The drawing under review shows one solid part. Ordinate dimensions are in mm from its lowest x, y, z. Give positions to 0.01 mm unless a question says otherwise; leave off trailing zeros. Loops run counter-clockwise (first coordinate to the right, second up) from the corner with the lowest first, then second, coordinate; pieces in that order, holes last. Notation, with made-up numbers: M 24.25,54 L 59.25,54 A6 cw 59.25,65 Z; hole C 9,31 d10. An arc over 180 degrees is marked long. One line per item, written item: value. Start each with the question number.
Q1. We need section B-B on y = 3.5. Write out the cut boundary in (x, z), plus the area to 3 significant figures.
Q2. For pin 1 (1.5 mm diameter, centred on y = 36.5, z = 30.5, fed in from -X); pin 2 (3 mm diameter, centred on x = 193.5, y = 40.5, fed in from -Z); pin 3 (1.6 mm diameter, centred on y = 44, z = 20.5, fed in from -X); pin 4 (12 mm diameter, centred on x = 66, z = 43, fed in from +Y), all flat-tipped, find the tip position at first contact; note any pin that passes through.
Q3. To check wall thickness, follow line 1 along Z through (x, y) = (13, 17.5); line 2 along X through (y, z) = (40.5, 23); line 3 along Y through (x, z) = (125.5, 16). State the ranges of each line that lie inside material, in increasing order. Write a range as from..to.
Q4. Mouldability with a two-part tool opening along X and no side actions: class the marked faces 1, 2 and 3 as released by +X, released by -X, zero draft, split by the parting line, or undercut.
Q5. We need section C-C on z = 21. Write out the cut boundary in (x, y).
Q6. We need section D-D on y = 45.5. Give the number of separate pieces and of enclosed holes in the cut face, plus the area to 3 significant figures.
Q7. We need section A-A on x = 192.5. Write out the cut boundary in (y, z).
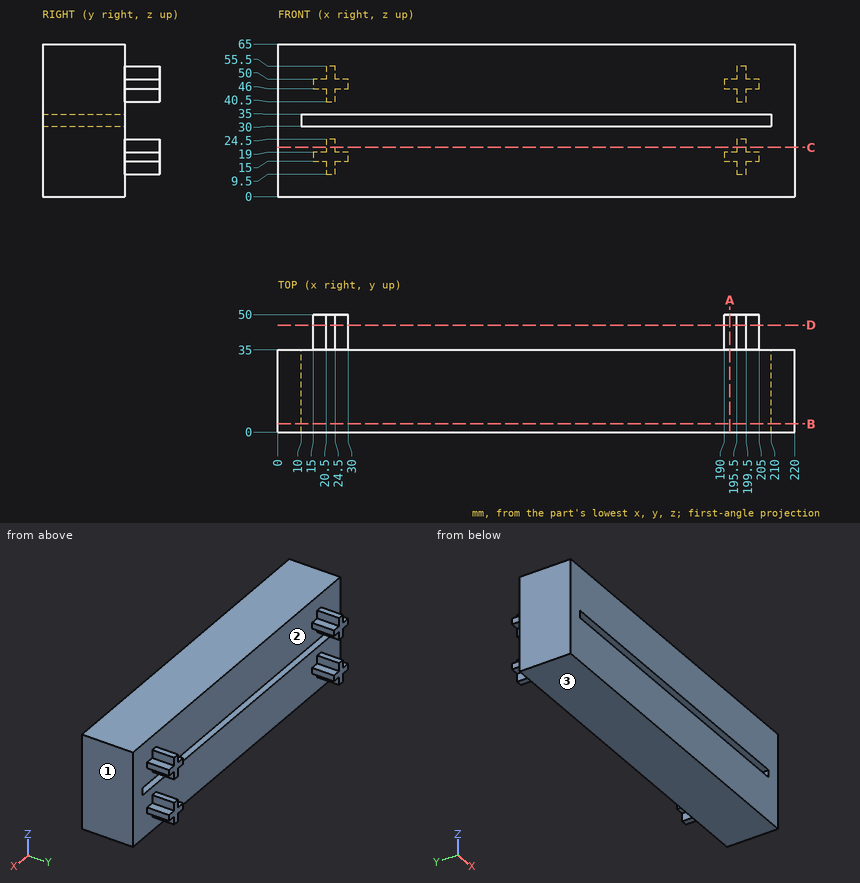
Solved:
1. outline: M 0,0 L 220,0 L 220,65 L 0,65 Z; hole M 10,30 L 210,30 L 210,35 L 10,35 Z
1. area: 13,300 mm2
2. pin 1: through
2. pin 2: z = 15
2. pin 3: x = 20.5
2. pin 4: y = 35
3. line 1: 0..30, 35..65
3. line 2: 20.5..24.5, 195.5..199.5
3. line 3: 0..35
4. face 1: released by +X
4. face 2: undercut
4. face 3: zero draft
5. outline: M 0,0 L 220,0 L 220,35 L 199.5,35 L 199.5,50 L 195.5,50 L 195.5,35 L 24.5,35 L 24.5,50 L 20.5,50 L 20.5,35 L 0,35 Z
6. separate pieces: 4
6. enclosed holes: 0
6. area: 416 mm2
7. outline: M 0,0 L 35,0 L 35,15 L 50,15 L 50,19 L 35,19 L 35,30 L 0,30 Z; M 0,35 L 35,35 L 35,46 L 50,46 L 50,50 L 35,50 L 35,65 L 0,65 Z
